from build123d import *

# Parameters (mm, degrees)
F0_R     = 31.5
F0_R_2   = 1.5
F0_R_3   = 6.25
F1_DEPTH = 13
F2_DEPTH = 13


# Not quite as in the source:
# - a feature names something its author has since deleted; it is built from what else it names


with BuildPart() as f1:
    # F0 (on Top) → F1 (new body)
    with BuildSketch(Plane.XY):
        Circle(F0_R)
        with BuildLine():
            ThreePointArc((1.2490459616, 15.951171875), (11.7470152674, 10.8631317909), (16, 0))
            ThreePointArc((16, 0), (15.6047795357, -3.5342404619), (14.4386430447, -6.8938804043))
            ThreePointArc((14.4386430447, -6.8938804043), (14.9265222791, -7.3539720324), (15.1064064606, -8))
            ThreePointArc((15.1064064606, -8), (14.4601399606, -9.0945345408), (13.1895970831, -9.0572914707))
            ThreePointArc((13.1895970831, -9.0572914707), (0, -16), (-13.1895970831, -9.0572914707))
            ThreePointArc((-13.1895970831, -9.0572914707), (-14.9389382153, -8.625), (-14.4386430447, -6.8938804043))
            ThreePointArc((-14.4386430447, -6.8938804043), (-13.8564064606, 8), (-1.2490459616, 15.951171875))
            ThreePointArc((-1.2490459616, 15.951171875), (-0.0244187222, 17.2497614676), (1.25, 16))
            ThreePointArc((1.25, 16), (1.2497614676, 15.9755812778), (1.2490459616, 15.951171875))
        make_face(mode=Mode.SUBTRACT)
        with BuildLine():
            ThreePointArc((14.4386430447, -6.8938804043), (15.6047795357, -3.5342404619), (16, 0))
            ThreePointArc((16, 0), (11.7470152674, 10.8631317909), (1.2490459616, 15.951171875))
            ThreePointArc((1.2490459616, 15.951171875), (0, 14.75), (-1.2490459616, 15.951171875))
            ThreePointArc((-1.2490459616, 15.951171875), (-13.8564064606, 8), (-14.4386430447, -6.8938804043))
            ThreePointArc((-14.4386430447, -6.8938804043), (-13.210378493, -6.9298841815), (-12.6064064606, -8))
            ThreePointArc((-12.6064064606, -8), (-12.7618719198, -8.6037335), (-13.1895970831, -9.0572914707))
            ThreePointArc((-13.1895970831, -9.0572914707), (0, -16), (13.1895970831, -9.0572914707))
            ThreePointArc((13.1895970831, -9.0572914707), (12.7738747058, -7.375), (14.4386430447, -6.8938804043))
        make_face()
        with Locations((-8.8388347648, -8.8388347648)):
            Circle(F0_R_2, mode=Mode.SUBTRACT)
        with Locations((8.8388347648, -8.8388347648)):
            Circle(F0_R_2, mode=Mode.SUBTRACT)
        with Locations((-8.8388347648, 8.8388347648)):
            Circle(F0_R_2, mode=Mode.SUBTRACT)
        Circle(F0_R_3, mode=Mode.SUBTRACT)
        with Locations((8.8388347648, 8.8388347648)):
            Circle(F0_R_2, mode=Mode.SUBTRACT)
    extrude(amount=F1_DEPTH)

    # F0 (on Top) → F2 (join)
    with BuildSketch(Plane.XY):
        Circle(F0_R)
        with BuildLine():
            ThreePointArc((1.2490459616, 15.951171875), (11.7470152674, 10.8631317909), (16, 0))
            ThreePointArc((16, 0), (15.6047795357, -3.5342404619), (14.4386430447, -6.8938804043))
            ThreePointArc((14.4386430447, -6.8938804043), (14.9265222791, -7.3539720324), (15.1064064606, -8))
            ThreePointArc((15.1064064606, -8), (14.4601399606, -9.0945345408), (13.1895970831, -9.0572914707))
            ThreePointArc((13.1895970831, -9.0572914707), (0, -16), (-13.1895970831, -9.0572914707))
            ThreePointArc((-13.1895970831, -9.0572914707), (-14.9389382153, -8.625), (-14.4386430447, -6.8938804043))
            ThreePointArc((-14.4386430447, -6.8938804043), (-13.8564064606, 8), (-1.2490459616, 15.951171875))
            ThreePointArc((-1.2490459616, 15.951171875), (-0.0244187222, 17.2497614676), (1.25, 16))
            ThreePointArc((1.25, 16), (1.2497614676, 15.9755812778), (1.2490459616, 15.951171875))
        make_face(mode=Mode.SUBTRACT)
        with BuildLine():
            ThreePointArc((14.4386430447, -6.8938804043), (15.6047795357, -3.5342404619), (16, 0))
            ThreePointArc((16, 0), (11.7470152674, 10.8631317909), (1.2490459616, 15.951171875))
            ThreePointArc((1.2490459616, 15.951171875), (0, 14.75), (-1.2490459616, 15.951171875))
            ThreePointArc((-1.2490459616, 15.951171875), (-13.8564064606, 8), (-14.4386430447, -6.8938804043))
            ThreePointArc((-14.4386430447, -6.8938804043), (-13.210378493, -6.9298841815), (-12.6064064606, -8))
            ThreePointArc((-12.6064064606, -8), (-12.7618719198, -8.6037335), (-13.1895970831, -9.0572914707))
            ThreePointArc((-13.1895970831, -9.0572914707), (0, -16), (13.1895970831, -9.0572914707))
            ThreePointArc((13.1895970831, -9.0572914707), (12.7738747058, -7.375), (14.4386430447, -6.8938804043))
        make_face()
        with Locations((-8.8388347648, -8.8388347648)):
            Circle(F0_R_2, mode=Mode.SUBTRACT)
        with Locations((8.8388347648, -8.8388347648)):
            Circle(F0_R_2, mode=Mode.SUBTRACT)
        with Locations((-8.8388347648, 8.8388347648)):
            Circle(F0_R_2, mode=Mode.SUBTRACT)
        Circle(F0_R_3, mode=Mode.SUBTRACT)
        with Locations((8.8388347648, 8.8388347648)):
            Circle(F0_R_2, mode=Mode.SUBTRACT)
        with BuildLine():
            ThreePointArc((-1.2490459616, 15.951171875), (0, 14.75), (1.2490459616, 15.951171875))
            ThreePointArc((1.2490459616, 15.951171875), (0, 16), (-1.2490459616, 15.951171875))
        make_face()
        with BuildLine():
            ThreePointArc((-1.2490459616, 15.951171875), (0, 16), (1.2490459616, 15.951171875))
            ThreePointArc((1.2490459616, 15.951171875), (1.2497614676, 15.9755812778), (1.25, 16))
            ThreePointArc((1.25, 16), (-0.0244187222, 17.2497614676), (-1.2490459616, 15.951171875))
        make_face()
        with BuildLine():
            ThreePointArc((15.1064064606, -8), (14.9265222791, -7.3539720324), (14.4386430447, -6.8938804043))
            ThreePointArc((14.4386430447, -6.8938804043), (13.8564064606, -8), (13.1895970831, -9.0572914707))
            ThreePointArc((13.1895970831, -9.0572914707), (14.4601399606, -9.0945345408), (15.1064064606, -8))
        make_face()
        with BuildLine():
            ThreePointArc((13.1895970831, -9.0572914707), (13.8564064606, -8), (14.4386430447, -6.8938804043))
            ThreePointArc((14.4386430447, -6.8938804043), (12.7738747058, -7.375), (13.1895970831, -9.0572914707))
        make_face()
        with BuildLine():
            ThreePointArc((-12.6064064606, -8), (-13.210378493, -6.9298841815), (-14.4386430447, -6.8938804043))
            ThreePointArc((-14.4386430447, -6.8938804043), (-13.8564064606, -8), (-13.1895970831, -9.0572914707))
            ThreePointArc((-13.1895970831, -9.0572914707), (-12.7618719198, -8.6037335), (-12.6064064606, -8))
        make_face()
        with BuildLine():
            ThreePointArc((-13.1895970831, -9.0572914707), (-13.8564064606, -8), (-14.4386430447, -6.8938804043))
            ThreePointArc((-14.4386430447, -6.8938804043), (-14.9389382153, -8.625), (-13.1895970831, -9.0572914707))
        make_face()
    extrude(amount=-F2_DEPTH)


solid = f1.part
Design review of the part built by this model. Coordinates are the model's own, in mm. A direction names the side the tool comes from. Round coordinates to 2 decimals unless told otherwise and drop trailing zeros. Order: outer loops, then holes, each group sorted by start corner. A loop starts at its lowest first (then second) coordinate and runs counter-clockwise, first axis right, second up.
1) Draft analysis for pull direction X (two halves, no side actions). For faces 3 (the flat face through (14, -8, 0)), 4 (the cylindrical face through (-4.101, 31.232, 0.182)), 5 (the flat face through (7, 0, 13)), state which applies: released by +X, released by -X, zero draft, split by the parting line, or undercut.
The answers:
face 3: undercut
face 4: split by the parting line
face 5: zero draft
2) Consider section D-D (x = 8.5). State the section outline as (y, z) points, plus the area to 3 significant figures.
The answers:
outline: (-30.33, -13) - (-10.3, -13) - (-10.3, 13) - (-30.33, 13) - close; (-7.38, -13) - (7.38, -13) - (7.38, 13) - (-7.38, 13) - close; (10.3, -13) - (30.33, -13) - (30.33, 13) - (10.3, 13) - close
area: 1,430 mm2
3) Consider section A-A (x = 0). State the section outline as (y, z) points.
The answers:
outline: (-31.5, -13) - (-6.25, -13) - (-6.25, 13) - (-31.5, 13) - close; (6.25, -13) - (31.5, -13) - (31.5, 13) - (17.25, 13) - (17.25, 0) - (14.75, 0) - (14.75, 13) - (6.25, 13) - close
4) Clearance check with flat-ended pins moving along their axes: pin 1 Ø1.2 at (x, y) = (13.5, -8) entering from +Z; pin 2 Ø5 at (y, z) = (9, -3.5) entering from -X; pin 3 Ø8 at (y, z) = (22.5, -8.5) entering from +X. State where each tip first meets the part, or that it passes through.
The answers:
pin 1: stops at z = 0
pin 2: stops at x = -30.82
pin 3: stops at x = 25.5
5) Consider section C-C (z = 7). Count the separate pieces of the cut face and the enclosed holes in it, plus the area to 3 significant figures.
The answers:
separate pieces: 1
enclosed holes: 8
area: 2,950 mm2
6) Machinability: for faces 1 (the cylindrical face through (-9.944, -7.825, -0.182)), 2 (the flat face through (-14, -8, 0)), which of the approach directions +Z, -Z, +X, -X, +Y, -Y give a long, thin tool a straight path to every point of the face, cutting with its end or side? Answer none if there is none.
The answers:
face 1: +Z, -Z
face 2: +Z
7) Consider section B-B (y = 0). State the section outline as (x, z) points.
The answers:
outline: (-31.5, -13) - (-6.25, -13) - (-6.25, 13) - (-31.5, 13) - close; (6.25, -13) - (31.5, -13) - (31.5, 13) - (6.25, 13) - close
8) For L1, parallel to X at y = 8, z = -0.5; L2, parallel to X at y = -10, z = -9.5; L3, parallel to X at y = -28, z = -0.75, list the stretches that pass through material, from the lowest coordinate up.
The answers:
L1: x = -30.47 to -10.08, -7.6 to 7.6, 10.08 to 30.47
L2: x = -29.87 to -9.79, -7.89 to 7.89, 9.79 to 29.87
L3: x = -14.43 to 14.43
